Read the model definition and answer for the solid it produces. Units are mm, in the model's axes. A direction names the side the tool comes from. Coordinates: 2 decimals unless noted, no trailing zeros. Write each loop counter-clockwise with the first axis right and the second up, starting at its lowest first coordinate (ties: lowest second). Pieces come first, ordered by that corner, then holes. Notation, with made-up numbers: (-35.75, 19) -> (-10.75, 19) arc R6 ccw to (-10.75, 29) -> close; hole circle Ø8 at (76, 1.25). An arc over 180 degrees is marked (long way). Return JSON: item names as keys, results as strings.
from build123d import *

# Parameters (mm, degrees)
SKETCH_1_R          = 1.5
SKETCH_1_R_2        = 1.6
EXTRUDE_1_DEPTH     = 5
CHAMFER_1_SIZE      = 2
SKETCH_2_R          = 2
CUT_EXTRUDE_1_DEPTH = 50.749371855
SKETCH_3_W          = 7.2
SKETCH_3_H          = 5.2
CUT_EXTRUDE_2_DEPTH = 40.449334595


with BuildPart() as part:
    # 草图1 → 凸台-拉伸1 (new body)
    with BuildSketch(Plane(origin=(0, 0, 0), x_dir=(1, 0, 0), z_dir=(0, 1, 0))):
        Polygon((35, 17.5), (-35, 17.5), (-35, 11.288596674), (-21.49999999, 11.288596674), (-21.49999999, -11.288596674), (-35, -11.288596674), (-35, -17.5), (35, -17.5), (35, -11.288596674), (21.49999999, -11.288596674), (21.49999999, 11.288596674), (35, 11.288596674), align=None)
        with Locations(Location((-28.303727501, -14.088596674, 0), (0, 0, 270))):
            Circle(SKETCH_1_R, mode=Mode.SUBTRACT)
        with Locations(Location((0, -10, 0), (0, 0, 270))):
            Circle(SKETCH_1_R_2, mode=Mode.SUBTRACT)
        with Locations(Location((28.303727501, -14.088596674, 0), (0, 0, 270))):
            Circle(SKETCH_1_R, mode=Mode.SUBTRACT)
        with Locations(Location((-28.303727501, 14.088596674, 0), (0, 0, 270))):
            Circle(SKETCH_1_R, mode=Mode.SUBTRACT)
        with Locations(Location((0, 5, 0), (0, 0, 270))):
            Circle(SKETCH_1_R_2, mode=Mode.SUBTRACT)
        with Locations(Location((28.303727501, 14.088596674, 0), (0, 0, 270))):
            Circle(SKETCH_1_R, mode=Mode.SUBTRACT)
    extrude(amount=EXTRUDE_1_DEPTH)

    # 倒角1
    chamfer_1_edges = [part.edges().sort_by_distance(p)[0] for p in [
        (35, 2.5, 11.288596674),
        (-35, 2.5, 11.288596674),
        (-35, 2.5, -11.288596674),
        (35, 2.5, -11.288596674),
    ]]
    chamfer(chamfer_1_edges, length=CHAMFER_1_SIZE)

    # 草图2 → 切除-拉伸1 (cut, through all)
    with BuildSketch(Plane.XY.offset(17.5)):
        with Locations((-15.8, 2.5)):
            Circle(SKETCH_2_R)
        with Locations(Location((15.8, 2.5, 0), (0, 0, 180))):
            Circle(SKETCH_2_R)
    extrude(amount=-CUT_EXTRUDE_1_DEPTH, mode=Mode.SUBTRACT)

    # 草图3 → 切除-拉伸2 (cut, through all)
    with BuildSketch(Plane(origin=(0, 5, 0), x_dir=(1, 0, 0), z_dir=(0, 1, 0))):
        with Locations((-15.8, 11.9)):
            Rectangle(SKETCH_3_W, SKETCH_3_H)
        with Locations((15.8, 11.9)):
            Rectangle(SKETCH_3_W, SKETCH_3_H)
    extrude(amount=-CUT_EXTRUDE_2_DEPTH, mode=Mode.SUBTRACT)


solid = part.part
1. For a pull along Y with two mould halves and no side action, classify faces 5 (the face through (35, 2, 15)), 6 (the face through (0, 0, 0)), 7 (the face through (0, 5, 0)), 8 (the face through (-17.4, 1.3, -16)) as +Y half, -Y half, draft (parallel to the pull), parting line (faces both ways), or undercut.
Taken from the geometry:
{"face 5": "draft", "face 6": "-Y half", "face 7": "+Y half", "face 8": "undercut"}
2. The part is cut by section B-B (x = -15.8). Determine the outline of the cut face in (y, z).
Taken from the geometry:
{"outline": "(0, -17.5) -> (0.5, -17.5) -> (0.5, -14.5) -> (0, -14.5) -> close; (0, -9.3) -> (0.5, -9.3) -> (0.5, 17.5) -> (0, 17.5) -> close; (4.5, -17.5) -> (5, -17.5) -> (5, -14.5) -> (4.5, -14.5) -> close; (4.5, -9.3) -> (5, -9.3) -> (5, 17.5) -> (4.5, 17.5) -> close"}
3. The part is cut by section A-A (z = -5). Determine the outline of the cut face in (x, y).
Taken from the geometry:
{"outline": "(-21.5, 0) -> (-1.6, 0) -> (-1.6, 5) -> (-21.5, 5) -> close; (1.6, 0) -> (21.5, 0) -> (21.5, 5) -> (1.6, 5) -> close; hole circle Ø4 at (-15.8, 2.5); hole circle Ø4 at (15.8, 2.5)"}
4. Consider L1, parallel to X at y = 2.45, z = 5; L2, parallel to Z at x = -32, y = 2.8; L3, parallel to Z at x = -18.5, y = 3.9. Determine where each line is inside the solid, lowest interval first.
Taken from the geometry:
{"L1": "x = -21.5 to -17.8, -13.8 to 13.8, 17.8 to 21.5", "L2": "z = -17.5 to -11.29, 11.29 to 17.5", "L3": "z = -17.5 to -14.5, -9.3 to 17.5"}
5. Flat-ended cylindrical pins translate along their axes: pin 1 Ø1 at (y, z) = (0.5, -10.5) entering from +X; pin 2 Ø1.5 at (y, z) = (1.5, -10.5) entering from -X; pin 3 Ø1.5 at (y, z) = (1.5, 11.5) entering from +X. Find the tip coordinate at first contact, or state that the pin passes through.
Taken from the geometry:
{"pin 1": "stops at x = 21.5", "pin 2": "stops at x = -21.5", "pin 3": "stops at x = 33.96"}
6. The part is cut by section D-D (y = 1.45). Count the separate pieces of the cut face and the enclosed holes in it, then the cut area to 3 significant figures.
Taken from the geometry:
{"separate pieces": "3", "enclosed holes": "6", "area": "1,510 mm2"}
7. A tool of negligible diameter and unlimited length cuts with its end or side. For faces 1 (the face through (27, 2, 11.289)), 2 (the face through (-35, 2, -15)), 3 (the face through (19.4, 3, -12)), 4 (the face through (-33.986, 2.465, -12.275)), from which of +Z, -Z, +X, -X, +Y, -Y can it reach the whole face along a straight path? Write none if from no direction.
Taken from the geometry:
{"face 1": "+X, +Y, -Y", "face 2": "+Z, -Z, -X, +Y, -Y", "face 3": "+Y, -Y", "face 4": "-X, +Y, -Y"}
8. The part is cut by section C-C (z = 14). Determine the outline of the cut face in (x, y).
Taken from the geometry:
{"outline": "(-35, 0) -> (-29.8, 0) -> (-29.8, 5) -> (-35, 5) -> close; (-26.81, 0) -> (26.81, 0) -> (26.81, 5) -> (-26.81, 5) -> close; (29.8, 0) -> (35, 0) -> (35, 5) -> (29.8, 5) -> close; hole circle Ø4 at (-15.8, 2.5); hole circle Ø4 at (15.8, 2.5)"}
